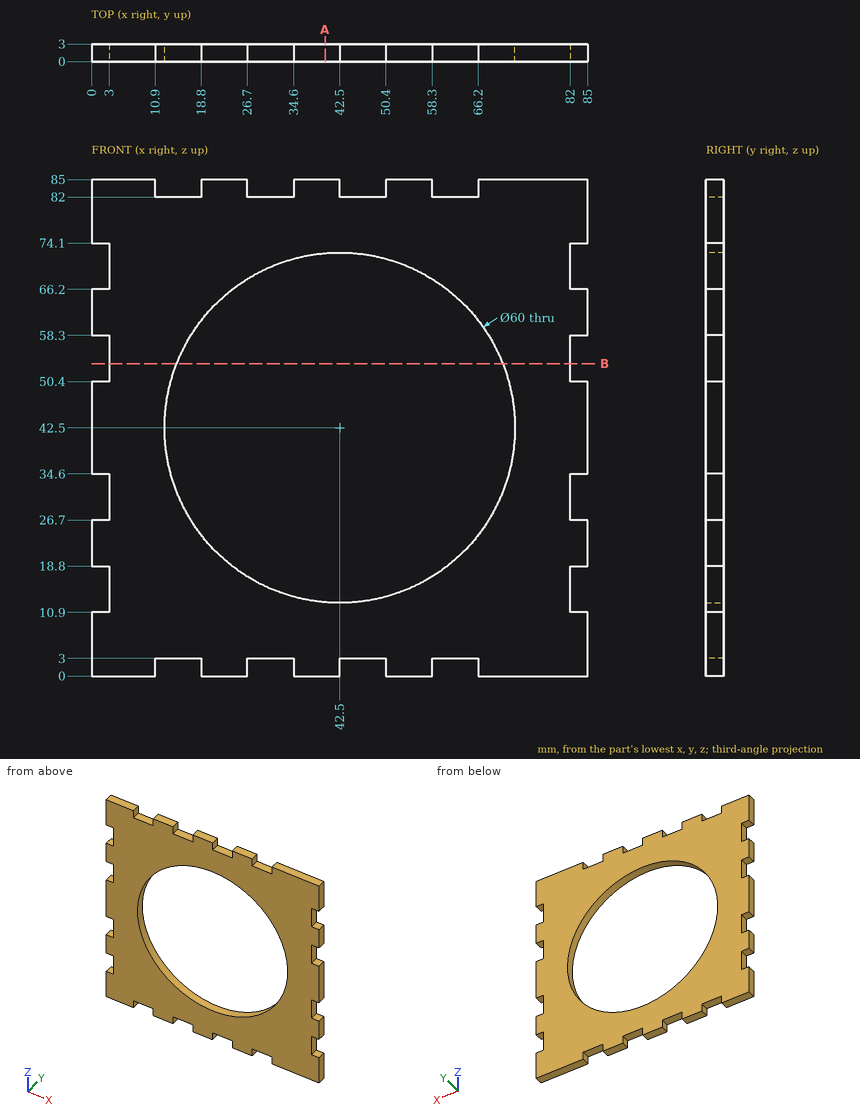
Job drawing, mm, ordinate dimensions from the low corner. One solid piece. Round coordinates to 2 decimals unless told otherwise and drop trailing zeros. Loops run counter-clockwise (first coordinate to the right, second up) from the corner with the lowest first, then second, coordinate; pieces in that order, holes last. Notation, with made-up numbers: M -10,-22 L 15,-22 A14 cw 15,2 Z; hole C 23,-31.75 d11. An arc over 180 degrees is marked long. Answer as CSV lines item,"result".
1. Wall check: probe 1 along X at (y, z) = (2.15, 42.5); probe 2 along X at (y, z) = (1, 17); probe 3 along Z at (x, y) = (27.5, 0.35). Give the ranges that are in metal, low to high. Write a range as [from, to].
Resolved:
probe 1,"x = [0, 12.5], [72.5, 85]"
probe 2,"x = [3, 26.7], [58.3, 82]"
probe 3,"z = [3, 16.52], [68.48, 82]"
2. Flat gauge pin, fed straight in: P1, Ø1.5, axis at y = 1, z = 29, coming from the +X side. Where does the tip first touch, or does it go through?
Resolved:
P1,"stops at x = 82"
3. Cut at A-A on x = 40. Write the cut outline in (y, z), then the cut area to 3 significant figures.
Resolved:
outline,"M 0,0 L 3,0 L 3,12.6 L 0,12.6 Z; M 0,72.4 L 3,72.4 L 3,85 L 0,85 Z"
area,"75.6 mm²"
4. Cut at B-B on z = 53.5. Write the cut outline in (x, y).
Resolved:
outline,"M 3,0 L 14.59,0 L 14.59,3 L 3,3 Z; M 70.41,0 L 82,0 L 82,3 L 70.41,3 Z"
